Input: part model. Units: mm. Frame: model coordinates. Face numbers are marked on the shaded views. A direction names the side the tool comes from. Coordinates: 2 decimals unless noted, no trailing zeros. Loops run counter-clockwise (first coordinate to the right, second up) from the corner with the lowest first, then second, coordinate; pieces in that order, holes last.
(1) Contact query for flat-ended pins moving along their axis: P1, Ø1, axis at y = 1.5, z = 2.5, coming from the -X side; P2, Ø1, axis at x = -3.5, y = 0, coming from the +Z side; P3, Ø3, axis at x = -4.49, y = 0, coming from the -Z side. Output: stop coordinate, or through.
(2) Line query: L1, parallel to Z at x = 6, y = 0; L2, parallel to X at y = 0, z = 0.5; L3, parallel to X at y = 0, z = 0.8. Output: solid intervals per line, ascending.
(3) Set-up query: the marked faces 1 and 2. Return all of +Z, -Z, +X, -X, +Y, -Y with unobstructed straight access to the full face (end or side cutting, diameter ignored); none if empty.
(4) Section A-A, the plane y = 0. Return loops of the section in (x, z), then the cut area to 3 significant figures.
(5) Section D-D, the plane x = 2.25. Return loops of the section in (y, z).
(6) Section B-B, the plane x = 10. Return loops of the section in (y, z).
(7) Section C-C, the plane y = 2.5. Return loops of the section in (x, z).
```python
from build123d import *

# Parameters (mm, degrees)
CHAMFER1_SIZE           = 0.5
SKETCH2_R               = 1
CUT_EXTRUDE1_DEPTH      = 4.5
CUT_EXTRUDE1_DEPTH_BACK = 4.5


with BuildPart() as part:
    # Sketch1 → Revolve1 (revolve)
    with BuildSketch(Plane.XY):
        with BuildLine():
            Line((-6.989590942, 0), (-6.989590942, 2))
            Line((-6.989590942, 2), (9.010409058, 2))
            Line((9.010409058, 2), (9.010409058, 3.5))
            ThreePointArc((9.010409058, 3.5), (11.485282792, 2.474873734), (12.510409058, 0))
            Line((12.510409058, 0), (-6.989590942, 0))
        make_face()
    revolve(axis=Axis((-10.070672023, 0, 0), (1, 0, 0)))

    # Chamfer1
    chamfer1_edges = [part.edges().sort_by_distance(p)[0] for p in [
        (-6.989590942, -2, 0),
    ]]
    chamfer(chamfer1_edges, length=CHAMFER1_SIZE)

    # Sketch2 → Cut-Extrude1 (cut, two sides)
    with BuildSketch(Plane.XY) as cut_extrude1_sk:
        with Locations((-4.489590942, 0)):
            Circle(SKETCH2_R)
    extrude(amount=CUT_EXTRUDE1_DEPTH, mode=Mode.SUBTRACT)
    extrude(cut_extrude1_sk.sketch, amount=-CUT_EXTRUDE1_DEPTH_BACK, mode=Mode.SUBTRACT)


solid = part.part
```
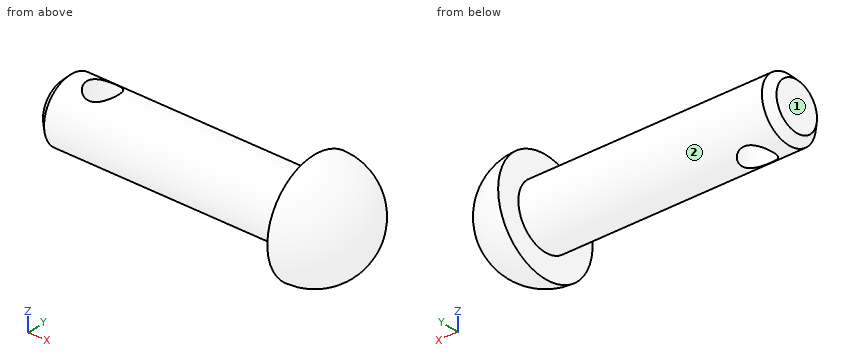
Report:
1. P1: stops at x = 9.01
1. P2: stops at z = 2
1. P3: stops at z = -2
2. L1: z = -2 to 2
2. L2: x = -6.99 to -5.49, -3.49 to 12.47
2. L3: x = -6.99 to -5.49, -3.49 to 12.42
3. face 1: +Z, -Z, -X, +Y, -Y
3. face 2: -X
4. outline: (-6.99, -1.5) - (-6.49, -2) - (-5.49, -2) - (-5.49, 2) - (-6.49, 2) - (-6.99, 1.5) - close; (-3.49, -2) - (9.01, -2) - (9.01, -3.5) arc R3.5 ccw to (9.01, 3.5) - (9.01, 2) - (-3.49, 2) - close
4. area: 75.0 mm2
5. outline: circle Ø4 at (0, 0)
6. outline: circle Ø6.71 at (0, 0)
7. outline: (9.01, -2.45) arc R2.45 ccw to (9.01, 2.45) - close
